Read the model definition and answer for the solid it produces. Units are mm, in the model's axes. Face numbers are marked on the shaded views. A direction names the side the tool comes from. Round coordinates to 2 decimals unless told otherwise and drop trailing zeros. Write each loop counter-clockwise with the first axis right and the second up, starting at its lowest first coordinate (ties: lowest second). Pieces come first, ordered by that corner, then holes. Notation, with made-up numbers: (27.5, 27) - (37.5, 27) arc R11 cw to (37.5, 31) - close; hole circle Ø2 at (87.5, -32). An arc over 180 degrees is marked (long way). Answer as CSV lines item,"result". Start each with the question number.
1) Find section C-C on z = -50. Determine the outline of the cut face in (x, y), then the cut area to 3 significant figures.
2) Find section B-B on x = 0. State how many separate pieces and enclosed holes the cut face has, then the cut area to 3 significant figures.
3) Each of these flat-tipped pins is pushed along its axis until it touches: pin 1 (5 mm diameter, centred on y = 7.5, z = -13, fed in from -X); pin 2 (8 mm diameter, centred on x = 17.66, z = -10.2, fed in from +Y); pin 3 (5.5 mm diameter, centred on x = 34.98, z = -20.2, fed in from +Y); pin 4 (1.5 mm diameter, centred on x = -30, y = 5.5, fed in from +Z). Where does it stop, or does it pass through?
4) Consider line 1 along X through (y, z) = (11.75, -10); line 2 along X through (y, z) = (6, -28); line 3 along Z through (x, y) = (40, 4.5). Determine where each line is inside the solid, lowest interval first.
5) For a pull along X with two mould halves and no side action, classify the marked faces 1, 2, 3 and 4 as +X half, -X half, draft (parallel to the pull), parting line (faces both ways), or undercut.
6) Which of the six approach directions +Z, -Z, +X, -X, +Y, -Y give full straight-line access (tool end or side, diameter ignored) to the marked faces 5 and 6?
7) Find section A-A on z = -70. Determine the outline of the cut face in (x, y).
from build123d import *

# Parameters (mm, degrees)
SKETCH1_R             = 7.5
SKETCH1_R_2           = 3
BOSS_EXTRUDE1_DEPTH   = 12.7
CROQUIS1_R            = 5.5
CORTAR_EXTRUIR1_DEPTH = 6


with BuildPart() as part:
    # Sketch1 → Boss-Extrude1 (new body)
    with BuildSketch(Plane(origin=(0, 0, 0), x_dir=(1, 0, 0), z_dir=(0, 1, 0))):
        with BuildLine():
            Line((5.692099788, 82.923700635), (18.827362954, 43.517911137))
            ThreePointArc((18.827362954, 43.517911137), (18.974757103, 40.242027017), (17.377903853, 37.377903853))
            Line((17.377903853, 37.377903853), (14.796225796, 34.796225796))
            ThreePointArc((14.796225796, 34.796225796), (13.683042429, 33.258238267), (13.106123272, 31.449441115))
            ThreePointArc((13.106123272, 31.449441115), (14.594879432, 28.035289019), (18.316890145, 27.895769532))
            Line((18.316890145, 27.895769532), (22.980762114, 30.588457268))
            ThreePointArc((22.980762114, 30.588457268), (25.980762114, 31.392304845), (28.980762114, 30.588457268))
            Line((28.980762114, 30.588457268), (37.980762114, 25.392304845))
            ThreePointArc((37.980762114, 25.392304845), (40.176914536, 23.196152423), (40.980762114, 20.196152423))
            Line((40.980762114, 20.196152423), (40.980762114, 9.803847577))
            ThreePointArc((40.980762114, 9.803847577), (40.176914536, 6.803847577), (37.980762114, 4.607695155))
            Line((37.980762114, 4.607695155), (33.316890145, 1.915007418))
            ThreePointArc((33.316890145, 1.915007418), (31.576712209, -1.378108157), (33.789076576, -4.374484859))
            ThreePointArc((33.789076576, -4.374484859), (35.644000439, -4.779256788), (37.532528394, -4.584205478))
            Line((37.532528394, -4.584205478), (41.059166204, -3.639245725))
            ThreePointArc((41.059166204, -3.639245725), (44.337996248, -3.688391827), (47.101298041, -5.453980963))
            Line((47.101298041, -5.453980963), (74.66008122, -36.5323473))
            ThreePointArc((74.66008122, -36.5323473), (75.367016076, -43.513167019), (68.967981432, -46.391353335))
            Line((68.967981432, -46.391353335), (28.273935087, -38.063930173))
            ThreePointArc((28.273935087, -38.063930173), (25.363239145, -36.55363519), (23.681262351, -33.738658128))
            Line((23.681262351, -33.738658128), (22.736302597, -30.212020318))
            ThreePointArc((22.736302597, -30.212020318), (21.960958009, -28.478981478), (20.682953305, -27.074956256))
            ThreePointArc((20.682953305, -27.074956256), (16.981832777, -26.657180862), (15, -29.81077695))
            Line((15, -29.81077695), (15, -35.196152423))
            ThreePointArc((15, -35.196152423), (14.196152423, -38.196152423), (12, -40.392304845))
            Line((12, -40.392304845), (3, -45.588457268))
            ThreePointArc((3, -45.588457268), (0, -46.392304845), (-3, -45.588457268))
            Line((-3, -45.588457268), (-12, -40.392304845))
            ThreePointArc((-12, -40.392304845), (-14.196152423, -38.196152423), (-15, -35.196152423))
            Line((-15, -35.196152423), (-15, -29.81077695))
            ThreePointArc((-15, -29.81077695), (-16.981832777, -26.657180862), (-20.682953305, -27.074956256))
            ThreePointArc((-20.682953305, -27.074956256), (-21.960958009, -28.478981478), (-22.736302597, -30.212020318))
            Line((-22.736302597, -30.212020318), (-23.681262351, -33.738658128))
            ThreePointArc((-23.681262351, -33.738658128), (-25.363239145, -36.55363519), (-28.273935087, -38.063930173))
            Line((-28.273935087, -38.063930173), (-68.967981432, -46.391353335))
            ThreePointArc((-68.967981432, -46.391353335), (-75.367016076, -43.51316702), (-74.66008122, -36.5323473))
            Line((-74.66008122, -36.5323473), (-47.101298041, -5.453980963))
            ThreePointArc((-47.101298041, -5.453980963), (-44.337996248, -3.688391827), (-41.059166204, -3.639245725))
            Line((-41.059166204, -3.639245725), (-37.532528394, -4.584205478))
            ThreePointArc((-37.532528394, -4.584205478), (-35.644000439, -4.779256788), (-33.789076576, -4.374484859))
            ThreePointArc((-33.789076576, -4.374484859), (-31.576712209, -1.378108157), (-33.316890145, 1.915007418))
            Line((-33.316890145, 1.915007418), (-37.980762114, 4.607695155))
            ThreePointArc((-37.980762114, 4.607695155), (-40.176914536, 6.803847577), (-40.980762114, 9.803847577))
            Line((-40.980762114, 9.803847577), (-40.980762114, 20.196152423))
            ThreePointArc((-40.980762114, 20.196152423), (-40.176914536, 23.196152423), (-37.980762114, 25.392304845))
            Line((-37.980762114, 25.392304845), (-28.980762114, 30.588457268))
            ThreePointArc((-28.980762114, 30.588457268), (-25.980762114, 31.392304845), (-22.980762114, 30.588457268))
            Line((-22.980762114, 30.588457268), (-18.316890145, 27.895769532))
            ThreePointArc((-18.316890145, 27.895769532), (-14.594879432, 28.035289019), (-13.106123272, 31.449441115))
            ThreePointArc((-13.106123272, 31.449441115), (-13.683042429, 33.258238267), (-14.796225796, 34.796225796))
            Line((-14.796225796, 34.796225796), (-17.377903853, 37.377903853))
            ThreePointArc((-17.377903853, 37.377903853), (-18.974757103, 40.242027017), (-18.827362954, 43.517911137))
            Line((-18.827362954, 43.517911137), (-5.692099788, 82.923700635))
            ThreePointArc((-5.692099788, 82.923700635), (0, 87.026334039), (5.692099788, 82.923700635))
        make_face()
        with Locations(Location((0, 0, 0), (0, 0, 270))):
            Circle(SKETCH1_R, mode=Mode.SUBTRACT)
        with Locations(Location((0, 70, 0), (0, 0, 270))):
            Circle(SKETCH1_R_2, mode=Mode.SUBTRACT)
        with Locations(Location((0, 50, 0), (0, 0, 270))):
            Circle(SKETCH1_R_2, mode=Mode.SUBTRACT)
        with Locations(Location((60.621778265, -35, 0), (0, 0, 270))):
            Circle(SKETCH1_R_2, mode=Mode.SUBTRACT)
        with Locations(Location((43.301270189, -25, 0), (0, 0, 270))):
            Circle(SKETCH1_R_2, mode=Mode.SUBTRACT)
        with Locations(Location((-60.621778265, -35, 0), (0, 0, 270))):
            Circle(SKETCH1_R_2, mode=Mode.SUBTRACT)
        with Locations(Location((-43.301270189, -25, 0), (0, 0, 270))):
            Circle(SKETCH1_R_2, mode=Mode.SUBTRACT)
        with Locations(Location((0, -40.392304845, 0), (0, 0, 270))):
            Circle(SKETCH1_R_2, mode=Mode.SUBTRACT)
        with Locations(Location((0, -20.392304845, 0), (0, 0, 270))):
            Circle(SKETCH1_R_2, mode=Mode.SUBTRACT)
        with Locations(Location((-34.980762114, 20.196152423, 0), (0, 0, 270))):
            Circle(SKETCH1_R_2, mode=Mode.SUBTRACT)
        with Locations(Location((-17.660254038, 10.196152423, 0), (0, 0, 270))):
            Circle(SKETCH1_R_2, mode=Mode.SUBTRACT)
        with Locations(Location((34.980762114, 20.196152423, 0), (0, 0, 270))):
            Circle(SKETCH1_R_2, mode=Mode.SUBTRACT)
        with Locations(Location((17.660254038, 10.196152423, 0), (0, 0, 270))):
            Circle(SKETCH1_R_2, mode=Mode.SUBTRACT)
    extrude(amount=BOSS_EXTRUDE1_DEPTH)

    # Croquis1 → Cortar-Extruir1 (cut)
    with BuildSketch(Plane.XZ):
        with Locations(Location((-60.621778265, 35, 0), (0, 0, 270))):
            Circle(CROQUIS1_R)
        with Locations(Location((-43.301270189, 25, 0), (0, 0, 270))):
            Circle(CROQUIS1_R)
        with Locations(Location((43.301270189, 25, 0), (0, 0, 270))):
            Circle(CROQUIS1_R)
        with Locations(Location((60.621778265, 35, 0), (0, 0, 270))):
            Circle(CROQUIS1_R)
        with Locations(Location((0, -50, 0), (0, 0, 270))):
            Circle(CROQUIS1_R)
        with Locations(Location((0, -70, 0), (0, 0, 270))):
            Circle(CROQUIS1_R)
    extrude(amount=-CORTAR_EXTRUIR1_DEPTH, mode=Mode.SUBTRACT)


solid = part.part
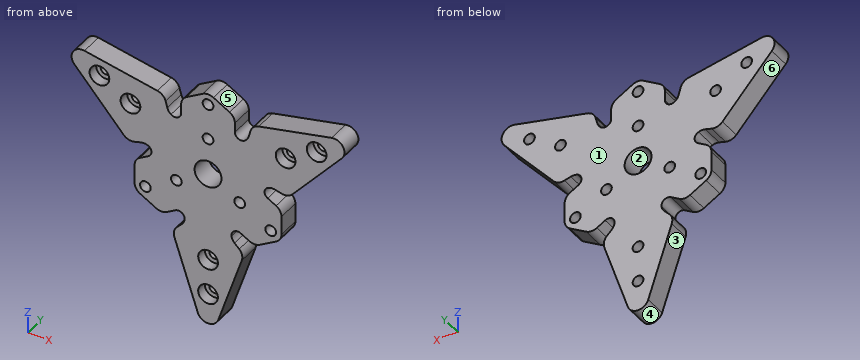
Check values:
1,outline,"(-16.67, 0) - (-5.5, 0) - (-5.5, 6) - (-3, 6) - (-3, 12.7) - (-16.67, 12.7) - close; (3, 6) - (5.5, 6) - (5.5, 0) - (16.67, 0) - (16.67, 12.7) - (3, 12.7) - close"
1,area,"317 mm^2"
2,separate pieces,"6"
2,enclosed holes,"0"
2,area,"1,140 mm^2"
3,pin 1,"stops at x = -40.98"
3,pin 2,"stops at y = 12.7"
3,pin 3,"passes through"
3,pin 4,"stops at z = 38.57"
4,line 1,"x = -40.98 to -20.65, -14.67 to 14.67, 20.65 to 40.98"
4,line 2,"x = -33.46 to -18.5, -14.65 to 14.65, 18.5 to 33.46"
4,line 3,"z = -23.48 to -6.52, 3.92 to 20.6, 29.4 to 40.46"
5,face 1,"draft"
5,face 2,"undercut"
5,face 3,"-X half"
5,face 4,"parting line"
6,face 5,"+Z, +Y, -Y"
6,face 6,"-Z, -X, +Y, -Y"
7,outline,"(-10, 0) - (-5.5, 0) - (-5.5, 6) - (-3, 6) - (-3, 12.7) - (-10, 12.7) - close; (3, 6) - (5.5, 6) - (5.5, 0) - (10, 0) - (10, 12.7) - (3, 12.7) - close"
